Design review of the part shown in the three views and the two pictorial views. Dimensions are in mm from the part's minimum x, y and z. Coordinates: 2 decimals unless noted, no trailing zeros. Loops run counter-clockwise (first coordinate to the right, second up) from the corner with the lowest first, then second, coordinate; pieces in that order, holes last. Notation, with made-up numbers: (57, 49.5) - (81, 49.5) arc R20 cw to (81, 64.5) - close; hole circle Ø5 at (60, 82). An arc over 180 degrees is marked (long way). One line per question, with ' | ' between items.
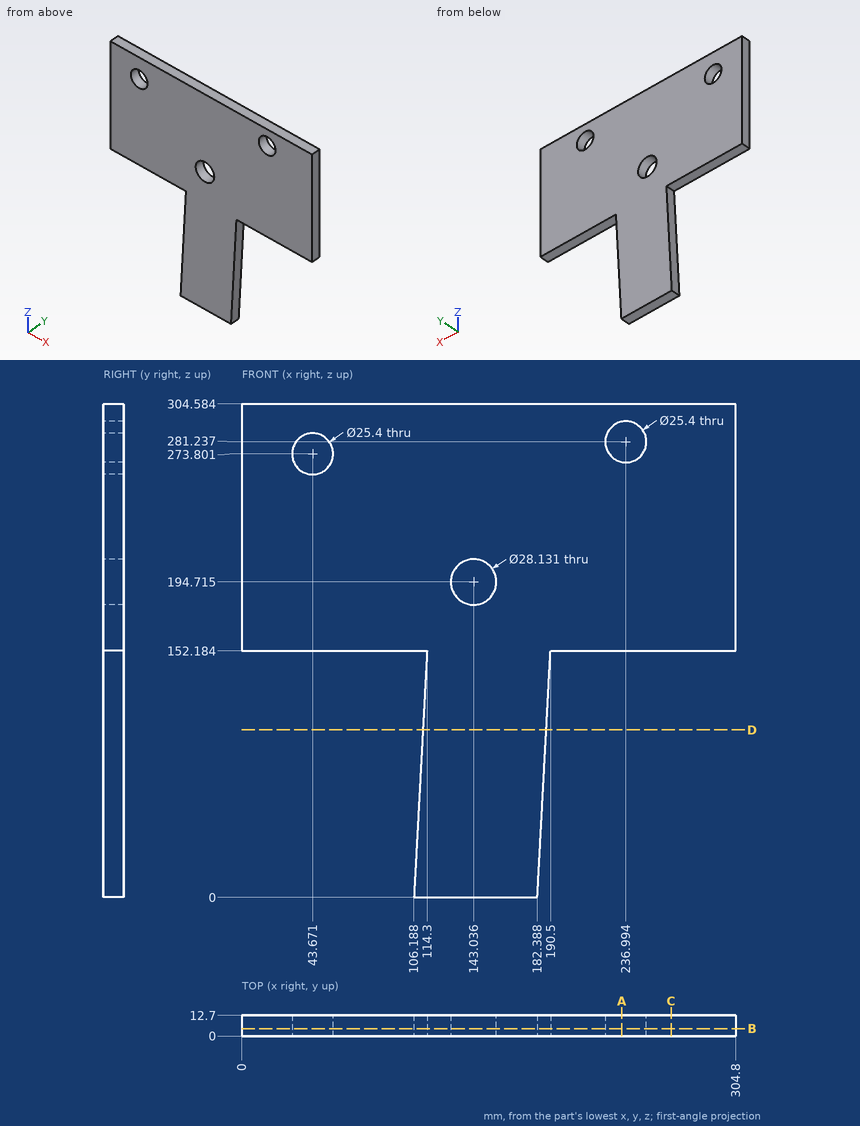
Q1. For pin 1 (17 mm diameter, centred on x = 143.04, z = 194.71, fed in from +Y); pin 2 (1 mm diameter, centred on x = 82.5, y = 11, fed in from -Z); pin 3 (3 mm diameter, centred on y = 10.5, z = 31, fed in from +X); pin 4 (1 mm diameter, centred on y = 5.5, z = 111, fed in from -X), all flat-tipped, find the tip position at first contact; note any pin that passes through.
Returned:
pin 1: passes through | pin 2: stops at z = 152.18 | pin 3: stops at x = 184.12 | pin 4: stops at x = 112.08
Q2. To check wall thickness, follow line 1 along Z through (x, y) = (43, 1.75) (1 decimal); line 2 along Z through (x, y) = (277.5, 2.25); line 3 along Z through (x, y) = (228.5, 1.75) (1 decimal). State the ranges of each line that lie inside material, in increasing order.
Returned:
line 1: z = 152.2 to 261.1, 286.5 to 304.6 | line 2: z = 152.18 to 304.58 | line 3: z = 152.2 to 271.8, 290.7 to 304.6
Q3. Take a section at A-A (x = 234.5). Give the boundary of the cut face in (y, z) (1 decimal).
Returned:
outline: (0, 152.2) - (12.7, 152.2) - (12.7, 268.8) - (0, 268.8) - close; (0, 293.7) - (12.7, 293.7) - (12.7, 304.6) - (0, 304.6) - close
Q4. Take a section at B-B (y = 4.5). Give the boundary of the cut face in (x, z) (1 decimal), plus the area to 3 significant figures.
Returned:
outline: (0, 152.2) - (114.3, 152.2) - (106.2, 0) - (182.4, 0) - (190.5, 152.2) - (304.8, 152.2) - (304.8, 304.6) - (0, 304.6) - close; hole circle Ø25.4 at (43.7, 273.8); hole circle Ø28.1 at (143, 194.7); hole circle Ø25.4 at (237, 281.2) | area: 56,400 mm²
Q5. Take a section at C-C (x = 265). Give the boundary of the cut face in (y, z).
Returned:
outline: (0, 152.18) - (12.7, 152.18) - (12.7, 304.58) - (0, 304.58) - close
Q6. Take a section at D-D (z = 103.5). Give the boundary of the cut face in (x, y) (1 decimal), plus the area to 3 significant figures.
Returned:
outline: (111.7, 0) - (187.9, 0) - (187.9, 12.7) - (111.7, 12.7) - close | area: 968 mm²
